Model file for the job. Use its own axes, mm. Face numbers are marked on the shaded views. A direction names the side the tool comes from. Round coordinates to 2 decimals unless told otherwise and drop trailing zeros. Order: outer loops, then holes, each group sorted by start corner. A loop starts at its lowest first (then second) coordinate and runs counter-clockwise, first axis right, second up. Notation, with made-up numbers: (61.25, 49.5) - (83.25, 49.5) arc R24 ccw to (83.25, 86.5) - close; hole circle Ø5 at (6.25, 77.25). An arc over 180 degrees is marked (long way). Use one line per item in the form item = value.
from build123d import *

# Parameters (mm, degrees)
F1_DEPTH = 15
F2_R     = 14.99999
F3_R     = 4.5
F4_DEPTH = 2.001
F5_R     = 10


# Not quite as in the source:
# - a fillet or chamfer is up to 0.001 mm smaller than in the source, because OpenCascade refuses the exact size


with BuildPart() as f1:
    # F0 (on Top) → F1 (new body, symmetric)
    with BuildSketch(Plane.XY):
        with BuildLine():
            ThreePointArc((-98.5355339059, -1.4644660941), (-100.15765065, -0.3806023374), (-102.0710678119, 0))
            Line((-102.0710678119, 0), (-140, 0))
            Line((-140, 0), (-140, -2))
            Line((-140, -2), (-102.8994949366, -2))
            ThreePointArc((-102.8994949366, -2), (-100.9860777748, -2.3806023374), (-99.3639610307, -3.4644660941))
            Line((-99.3639610307, -3.4644660941), (-78.4644660941, -24.3639610307))
            ThreePointArc((-78.4644660941, -24.3639610307), (-77.3806023374, -25.9860777748), (-77, -27.8994949366))
            Line((-77, -27.8994949366), (-77, -55))
            Line((-77, -55), (-75, -55))
            Line((-75, -55), (-75, -27.0710678119))
            ThreePointArc((-75, -27.0710678119), (-75.3806023374, -25.15765065), (-76.4644660941, -23.5355339059))
            Line((-76.4644660941, -23.5355339059), (-98.5355339059, -1.4644660941))
        make_face()
    extrude(amount=F1_DEPTH, both=True)

    # F2 (radius 15 in the source; OpenCascade refuses exactly that, so slightly less here)
    f2_edges = [f1.edges().sort_by_distance(p)[0] for p in [
        (-76, -55, 15),
        (-76, -55, -15),
    ]]
    fillet(f2_edges, radius=F2_R)

    # F3 (on face) → F4 (cut, through all)
    with BuildSketch(Plane.XZ.offset(2)):
        with Locations((-125, 0)):
            Circle(F3_R)
    extrude(amount=-F4_DEPTH, mode=Mode.SUBTRACT)

    # F5
    f5_edges = [f1.edges().sort_by_distance(p)[0] for p in [
        (-140, -1, 15),
        (-140, -1, -15),
    ]]
    fillet(f5_edges, radius=F5_R)


solid = f1.part
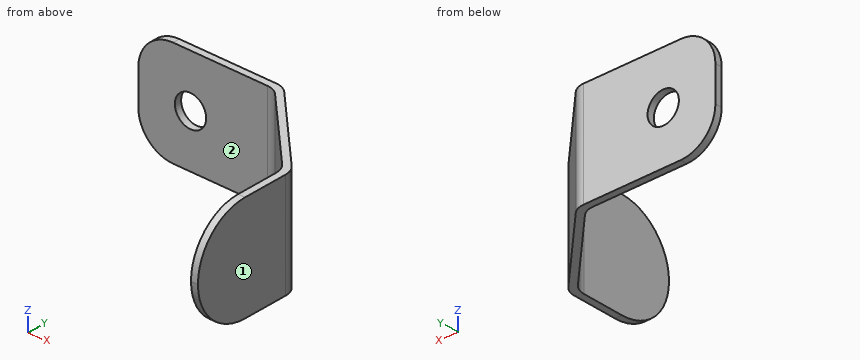
(1) Slice it at C-C on z = -11. Give the cut face in (x, y), then the cut area to 3 significant figures.
Report:
outline = (-138, -2) - (-102.9, -2) arc R5 cw to (-99.36, -3.46) - (-78.46, -24.36) arc R5 cw to (-77, -27.9) - (-77, -50.2) - (-75, -50.2) - (-75, -27.07) arc R5 ccw to (-76.46, -23.54) - (-98.54, -1.46) arc R5 ccw to (-102.07, 0) - (-138, 0) - close
area = 194 mm2
(2) Slice it at B-B on z = -2. Give the cut face in (x, y).
Report:
outline = (-140, -2) - (-129.03, -2) - (-129.03, 0) - (-140, 0) - close; (-120.97, -2) - (-102.9, -2) arc R5 cw to (-99.36, -3.46) - (-78.46, -24.36) arc R5 cw to (-77, -27.9) - (-77, -54.87) - (-75, -54.87) - (-75, -27.07) arc R5 ccw to (-76.46, -23.54) - (-98.54, -1.46) arc R5 ccw to (-102.07, 0) - (-120.97, 0) - close
(3) Probe probe 1 along Z at (x, y) = (-125, -1.2); probe 2 along Y at (x, z) = (-128.5, 13.5); probe 3 along X at (y, z) = (-31, -4.5). List the from-to ranges inside material, lowest first. Write a range as [from, to].
Report:
probe_1 = [-15, -4.5], [4.5, 15]
probe_2 = [-2, 0]
probe_3 = [-77, -75]
(4) Tool access for the marked faces 1 and 2: list every direction of +Z, -Z, +X, -X, +Y, -Y with a clear straight run to the whole face (end or side of a thin tool).
Report:
face_1 = +Z, -Z, +X, +Y, -Y
face_2 = +Z, -Z, -X, -Y
(5) Pin check, flat tips, straight feed: pin 1 (9 mm diameter, centred on x = -128.5, z = 7, fed in from -Y); pin 2 (3 mm diameter, centred on y = -7, z = 3, fed in from -X); pin 3 (3 mm diameter, centred on x = -92, y = -11, fed in from +Z); pin 4 (1 mm diameter, centred on x = -97, z = -5, fed in from +Y). Stop position of each tip, or through.
Report:
pin_1 = -2
pin_2 = -97.33
pin_3 = 15
pin_4 = -2.5
(6) Slice it at A-A on x = -125. Give the cut face in (y, z), then the cut area to 3 significant figures.
Report:
outline = (-2, -15) - (0, -15) - (0, -4.5) - (-2, -4.5) - close; (-2, 4.5) - (0, 4.5) - (0, 15) - (-2, 15) - close
area = 42.0 mm2
(7) Slice it at D-D on x = -86.5. Give the cut face in (y, z).
Report:
outline = (-16.33, -15) - (-13.5, -15) - (-13.5, 15) - (-16.33, 15) - close
